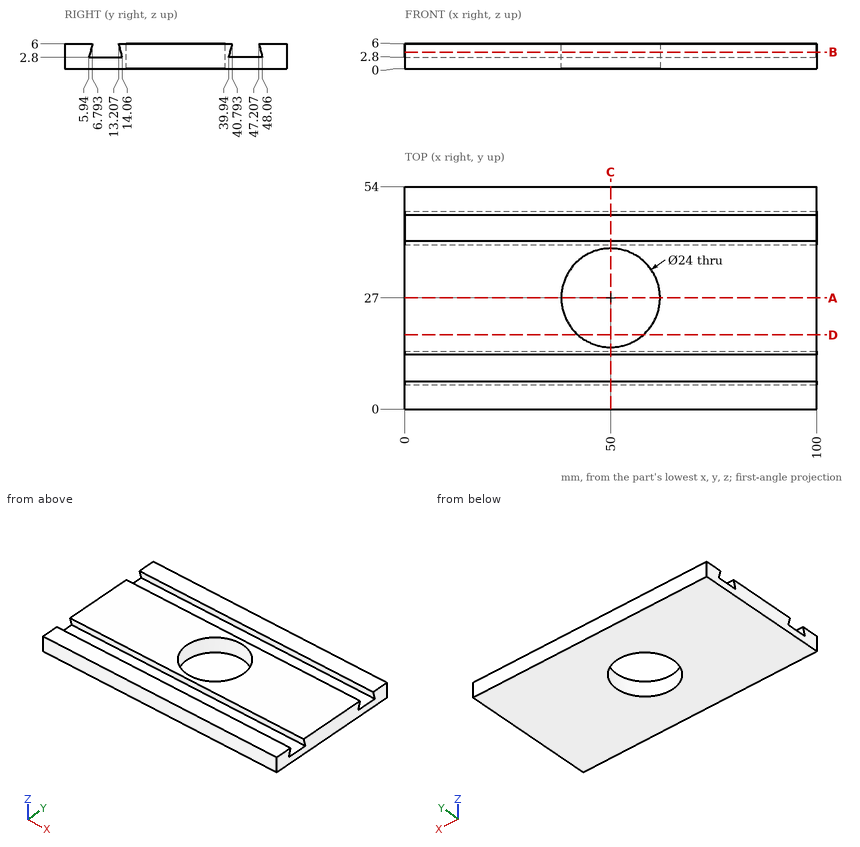
Here's the drawing with two shaded views (mm, measured from the low corner). I have some questions. Give positions to 0.01 mm unless a question says otherwise; leave off trailing zeros. Loops run counter-clockwise (first coordinate to the right, second up) from the corner with the lowest first, then second, coordinate; pieces in that order, holes last. Notation, with made-up numbers: (28.25, -33) -> (76.25, -33) arc R27 cw to (76.25, -10) -> close; hole circle Ø7 at (-18.75, 53.5). An arc over 180 degrees is marked (long way). One line per item, written item: value.
Q1. Suppose I cut it at D-D on y = 18. Please give me the cut outline in (x, z).
Answers follow:
outline: (0, 0) -> (42.06, 0) -> (42.06, 6) -> (0, 6) -> close; (57.94, 0) -> (100, 0) -> (100, 6) -> (57.94, 6) -> close
Q2. If I drill on line 1 along Y through (x, z) = (50, 2.25); line 2 along Y through (x, z) = (85, 5.35); line 3 along Y through (x, z) = (50, 4.8), over which ranges is the centre line in solid material (lowest first)?
Answers follow:
line 1: 0 to 15, 39 to 54
line 2: 0 to 6.62, 13.38 to 40.62, 47.38 to 54
line 3: 0 to 6.47, 13.53 to 15, 39 to 40.47, 47.53 to 54
Q3. Suppose I cut it at C-C on x = 50. Please give me the cut outline in (y, z).
Answers follow:
outline: (0, 0) -> (15, 0) -> (15, 6) -> (13.21, 6) -> (14.06, 2.8) -> (5.94, 2.8) -> (6.79, 6) -> (0, 6) -> close; (39, 0) -> (54, 0) -> (54, 6) -> (47.21, 6) -> (48.06, 2.8) -> (39.94, 2.8) -> (40.79, 6) -> (39, 6) -> close
Q4. Suppose I cut it at B-B on z = 4.05. Please give me the cut outline in (x, y).
Answers follow:
outline: (0, 0) -> (100, 0) -> (100, 6.27) -> (0, 6.27) -> close; (0, 13.73) -> (100, 13.73) -> (100, 40.27) -> (0, 40.27) -> close; (0, 47.73) -> (100, 47.73) -> (100, 54) -> (0, 54) -> close; hole circle Ø24 at (50, 27)
Q5. I'm going to push a flat-ended pin straight in: pin 1 Ø2.5 at (x, y) = (31.5, 43) entering from +Z. Where does the tip first touch, or does it pass through?
Answers follow:
pin 1: z = 2.8
Q6. Suppose I cut it at A-A on y = 27. Please give me the cut outline in (x, z).
Answers follow:
outline: (0, 0) -> (38, 0) -> (38, 6) -> (0, 6) -> close; (62, 0) -> (100, 0) -> (100, 6) -> (62, 6) -> close
